Autodesk Inventor part; units mm, degrees
ref_plane "YZ Plane" through (0, 0, 0) normal (1, 0, 0) x (0, 1, 0)
ref_plane "XZ Plane" through (0, 0, 0) normal (0, 1, 0) x (-1, 0, 0)
ref_plane "XY Plane" through (0, 0, 0) normal (0, 0, 1) x (1, 0, 0)
sketch "스케치1" plane through (0, 0, 0) normal (0, 0, 1) x (1, 0, 0)
  line L0 (-16.5, 8.6) -> (16.5, 8.6)
  line L1 (16.5, 8.6) -> (16.5, -8.6)
  line L2 (16.5, -8.6) -> (-16.5, -8.6)
  line L3 (-16.5, -8.6) -> (-16.5, 8.6)
  line L4 (-16.5, 8.6) -> (16.5, -8.6) construction
  line L5 (16.5, 8.6) -> (-16.5, -8.6) construction
  line L6 (13.52, 6.8) -> (14.42, 6.8)
  line L7 (14.42, 6.8) -> (14.42, 5.9)
  line L8 (14.42, 5.9) -> (13.52, 5.9)
  line L9 (13.52, 5.9) -> (13.52, 6.8)
  line L10 (13.52, 6.8) -> (14.42, 5.9) construction
  line L11 (14.42, 6.8) -> (13.52, 5.9) construction
  line L12 (13.52, -5.9) -> (14.42, -5.9)
  line L13 (14.42, -5.9) -> (14.42, -6.8)
  line L14 (14.42, -6.8) -> (13.52, -6.8)
  line L15 (13.52, -6.8) -> (13.52, -5.9)
  line L16 (13.52, -5.9) -> (14.42, -6.8) construction
  line L17 (14.42, -5.9) -> (13.52, -6.8) construction
  line L18 (-14.42, 3.36) -> (-13.52, 3.36)
  line L19 (-13.52, 3.36) -> (-13.52, 4.26)
  line L20 (-13.52, 4.26) -> (-14.42, 4.26)
  line L21 (-14.42, 4.26) -> (-14.42, 3.36)
  line L22 (-14.42, 3.36) -> (-13.52, 4.26) construction
  line L23 (-13.52, 3.36) -> (-14.42, 4.26) construction
  line L24 (-14.42, -3.36) -> (-13.52, -3.36)
  line L25 (-13.52, -3.36) -> (-13.52, -4.26)
  line L26 (-13.52, -4.26) -> (-14.42, -4.26)
  line L27 (-14.42, -4.26) -> (-14.42, -3.36)
  line L28 (-14.42, -3.36) -> (-13.52, -4.26) construction
  line L29 (-13.52, -3.36) -> (-14.42, -4.26) construction
  point P0 (0, 0)
  point P1 (13.97, 6.35)
  point P2 (13.97, -6.35)
  point P3 (-13.97, 3.81)
  point P4 (-13.97, -3.81)
  dimension "d0" = 33
  dimension "d1" = 17.2
  dimension "d2" = 2.25
  dimension "d3" = 12.7
  dimension "d4" = 0.9
  dimension "d5" = 0.9
  dimension "d6" = 0.9
  dimension "d7" = 0.9
  dimension "d8" = 0.9
  dimension "d9" = 0.9
  dimension "d10" = 0.9
  dimension "d11" = 0.9
  dimension "d12" = 4.79
  dimension "d13" = 7.62
  dimension "d14" = 2.53
  dimension "d15" = 27.94
extrude "돌출1" add sketch "스케치1" against normal blind 16.8 contours L0 L1 L2 L3 | L6 L7 L8 L9 | L12 L13 L14 L15 | L21 L20 L19 L18 | L24 L25 L26 L27
extrude "돌출2" add sketch "스케치1" along normal blind 10 contours L6 L7 L8 L9 | L12 L13 L14 L15 | L21 L20 L19 L18 | L24 L25 L26 L27
properties part number "GMS0205"
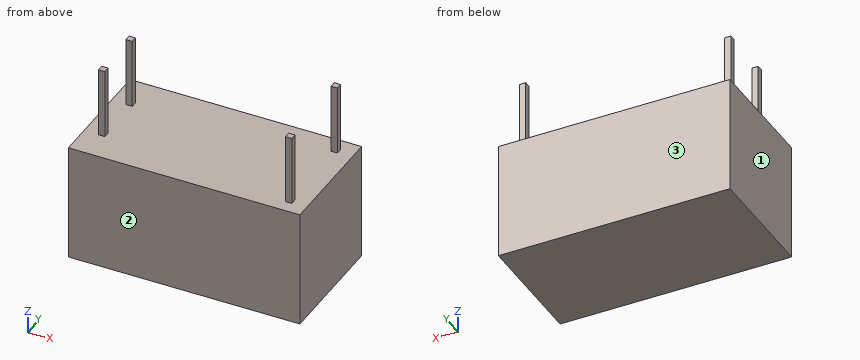
CAD build for the part. Positions are in the model's coordinates, mm. Face numbers are marked on the shaded views. Coordinates: 2 decimals unless noted, no trailing zeros. Order: outer loops, then holes, each group sorted by start corner. A loop starts at its lowest first (then second) coordinate and runs counter-clockwise, first axis right, second up. Notation, with made-up numbers: (85, -12) - (112, -12) arc R29 ccw to (112, 20) - close; hole circle Ø11 at (28, 43). An arc over 180 degrees is marked (long way). Answer in a Markdown table with one row per item.
1. Slice it at C-C, the plane y = -7.25. List the corners of the cut face in (x, z).
Answer:
| item | result |
|---|---|
| outline | (-16.5, -16.8) - (16.5, -16.8) - (16.5, 0) - (-16.5, 0) - close |
2. Slice it at A-A, the plane z = 4.5. List the corners of the cut face in (x, y), then the cut area to 3 significant figures.
Answer:
| item | result |
|---|---|
| outline | (-14.42, -4.26) - (-13.52, -4.26) - (-13.52, -3.36) - (-14.42, -3.36) - close; (-14.42, 3.36) - (-13.52, 3.36) - (-13.52, 4.26) - (-14.42, 4.26) - close; (13.52, -6.8) - (14.42, -6.8) - (14.42, -5.9) - (13.52, -5.9) - close; (13.52, 5.9) - (14.42, 5.9) - (14.42, 6.8) - (13.52, 6.8) - close |
| area | 3.24 mm² |
3. Drill centre lines: L1, parallel to Y at x = -14, z = 1; L2, parallel to Z at x = 4.5, y = -3; L3, parallel to X at y = -6.5, z = 6.5. Where is each one in solid material? Low to high. Write a range as from..to.
Answer:
| item | result |
|---|---|
| L1 | -4.26..-3.36, 3.36..4.26 |
| L2 | -16.8..0 |
| L3 | 13.52..14.42 |
4. Slice it at B-B, the plane x = 6. List the corners of the cut face in (y, z).
Answer:
| item | result |
|---|---|
| outline | (-8.6, -16.8) - (8.6, -16.8) - (8.6, 0) - (-8.6, 0) - close |
5. Flat gauge pins, fed straight in: P1, Ø1, axis at y = -4, z = 5.5, coming from the -X side; P2, Ø0.5, axis at x = 14, z = 6, coming from the -Y side; P3, Ø0.5, axis at x = -14, z = 5.5, coming from the -Y side. Where does each tip first touch, or does it go through?
Answer:
| item | result |
|---|---|
| P1 | x = -14.42 |
| P2 | y = -6.8 |
| P3 | y = -4.26 |
6. Pull direction Y, two halves, no side cores. Call the marked faces 1, 2 and 3: +Y half, -Y half, draft (parallel to the pull), parting line (faces both ways), or undercut.
Answer:
| item | result |
|---|---|
| face 1 | draft |
| face 2 | -Y half |
| face 3 | +Y half |
